Could you check a few things on this drawing? It's one solid part, dimensions in mm from its lowest x, y, z. A direction names the side the tool comes from. Give positions to 0.01 mm unless a question says otherwise; leave off trailing zeros. Loops run counter-clockwise (first coordinate to the right, second up) from the corner with the lowest first, then second, coordinate; pieces in that order, holes last. Notation, with made-up numbers: (89.25, -34) -> (123.25, -34) arc R28 cw to (123.25, -1) -> close; hole circle Ø11 at (-38, 66.5). An arc over 180 degrees is marked (long way). Use CSV: the item, a comma, the result in double quotes.
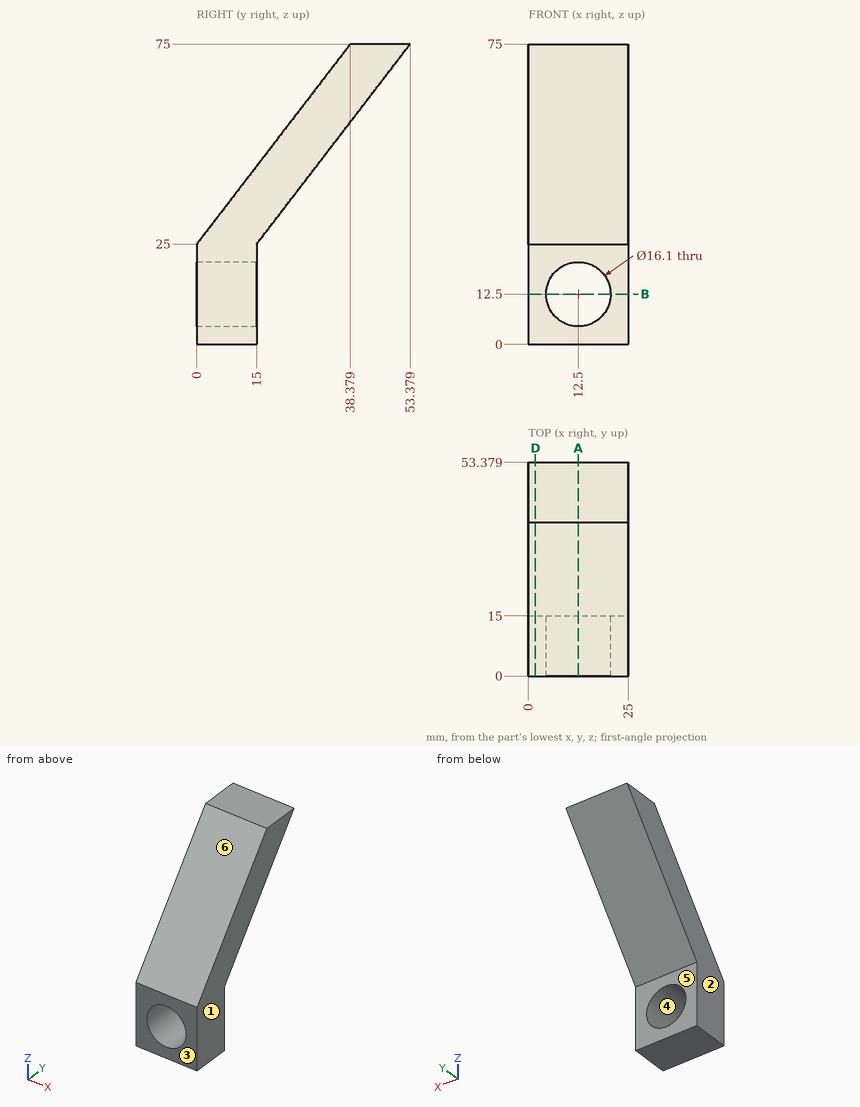
(1) If we section it at D-D, the plane x = 1.75: Write out the boundary of the cut face in (y, z).
Answer sheet:
outline,"(0, 0) -> (15, 0) -> (15, 25) -> (53.38, 75) -> (38.38, 75) -> (0, 25) -> close"
(2) If I drill on L1, parallel to X at y = 6.5, z = 12.5; L2, parallel to Z at x = 18, y = 8.5 (1 decimal); L3, parallel to Z at x = 16.75, y = 5 (1 decimal), over which ranges is the centre line in solid material (lowest first)? Write a range as from..to.
Answer sheet:
L1,"x = 0..4.45, 20.55..25"
L2,"z = 0..6.6, 18.4..36.1"
L3,"z = 0..5.7, 19.3..31.5"
(3) If we section it at A-A, the plane x = 12.5: Write out the boundary of the cut face in (y, z).
Answer sheet:
outline,"(0, 0) -> (15, 0) -> (15, 4.45) -> (0, 4.45) -> close; (0, 20.55) -> (15, 20.55) -> (15, 25) -> (53.38, 75) -> (38.38, 75) -> (0, 25) -> close"
(4) If we section it at B-B, the plane z = 12.5: Write out the boundary of the cut face in (x, y).
Answer sheet:
outline,"(0, 0) -> (4.45, 0) -> (4.45, 15) -> (0, 15) -> close; (20.55, 0) -> (25, 0) -> (25, 15) -> (20.55, 15) -> close"
(5) Which directions (+Z, -Z, +X, -X, +Y, -Y) give clear straight access to the entire face, cutting with the end or side of a thin tool? Please do the marked faces 5 and 6.
Answer sheet:
face 5,"-Z, +X, -X, +Y"
face 6,"+Z, +X, -X, -Y"
(6) Will these pins go through, and if not, where does the flat tip stop? pin 1 Ø6 at (x, z) = (9, 22.5) entering from +Y; pin 2 Ø2 at (x, y) = (7.5, 16.5) entering from -Z; pin 3 Ø4 at (x, z) = (21, 52.5) entering from +Y.
Answer sheet:
pin 1,"stops at y = 15.38"
pin 2,"stops at z = 25.65"
pin 3,"stops at y = 37.64"
(7) We'd pull the mould along X, two halves only. Please class the marked faces 1, 2, 3 and 4: released by +X, released by -X, zero draft, split by the parting line, or undercut.
Answer sheet:
face 1,"released by +X"
face 2,"released by -X"
face 3,"zero draft"
face 4,"undercut"
